Here's how the part is built. I have some questions about the finished solid (model axes, mm). Give positions to 0.01 mm unless a question says otherwise; leave off trailing zeros. Write each loop counter-clockwise with the first axis right and the second up, starting at its lowest first coordinate (ties: lowest second). Pieces come first, ordered by that corner, then holes. Notation, with made-up numbers: M 24,-30.75 L 75,-30.75 A10 cw 75,-15.75 Z; hole C 89.5,59 d7. An arc over 180 degrees is marked long. Answer as CSV lines item,"result". Start each with the question number.
Q1. For pin 1 (3 mm diameter, centred on x = 15.5, z = 490.5, fed in from -Y); pin 2 (2 mm diameter, centred on x = 16.5, z = 474.5, fed in from -Y); pin 3 (1.5 mm diameter, centred on x = 15.5, z = 470.5, fed in from -Y), each with a flat end and sliding along its axis, tell me the tip position at first contact or that it passes through.
Q2. Suppose I cut it at C-C (z = 475). Write out the boundary of the cut face in (x, y).
Q3. If I drill on line 1 along Y through (x, z) = (14.5, 498); line 2 along Y through (x, z) = (12.7, 466); line 3 along Z through (x, y) = (14.2, 2.5), over which ranges is the centre line in solid material (lowest first)?
Q4. Suppose I cut it at A-A (z = 469). Write out the boundary of the cut face in (x, y), then the cut area to 3 significant figures.
Q5. Suppose I cut it at B-B (x = 14.55). Write out the boundary of the cut face in (y, z), then the cut area to 3 significant figures.
Q6. Suppose I cut it at D-D (y = 19). Write out the boundary of the cut face in (x, z).
```python
from build123d import *

# Parameters (mm, degrees)
SKETCH1_R           = 2.2
SKETCH1_R_2         = 1.7
BOSS_EXTRUDE1_DEPTH = 5.08


with BuildPart() as part:
    # Sketch1 → Boss-Extrude1 (new body)
    with BuildSketch(Plane(origin=(17.497777778, 0, 0), x_dir=(0, 0, -1), z_dir=(1, 0, 0))):
        with BuildLine():
            Line((-499.600738517, 24.004018568), (-470.286926412, -0.333409807))
            ThreePointArc((-470.286926412, -0.333409807), (-464.654250247, 0.189045178), (-465.176705231, 5.821721344))
            Line((-465.176705231, 5.821721344), (-494.490517336, 30.159149718))
            ThreePointArc((-494.490517336, 30.159149718), (-500.123193502, 29.636694733), (-499.600738517, 24.004018568))
        make_face()
        with Locations((-467.731815822, 2.744155769)):
            Circle(SKETCH1_R, mode=Mode.SUBTRACT)
        with Locations((-497.045627927, 27.081584143)):
            Circle(SKETCH1_R_2, mode=Mode.SUBTRACT)
    extrude(amount=-BOSS_EXTRUDE1_DEPTH)


solid = part.part
```
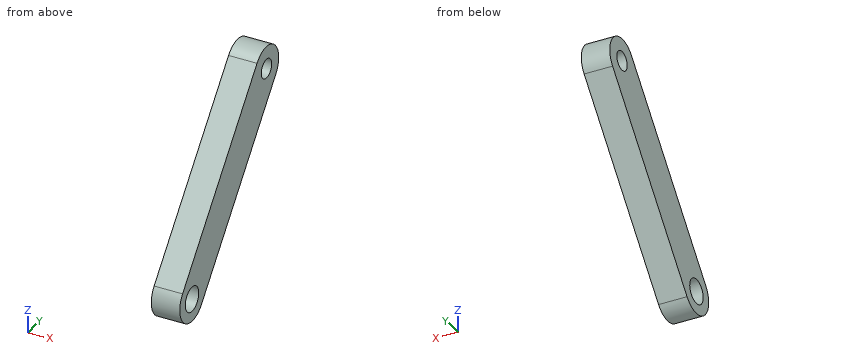
Resolved:
1,pin 1,"y = 15.2"
1,pin 2,"y = 2.33"
1,pin 3,"y = -0.71"
2,outline,"M 12.42,3.58 L 17.5,3.58 L 17.5,13.98 L 12.42,13.98 Z"
3,line 1,"22.68 to 25.67, 28.49 to 30.97"
3,line 2,"-0.86 to 1.39, 4.1 to 6.51"
3,line 3,"463.74 to 465.55, 469.92 to 473.7"
4,outline,"M 12.42,-1.05 L 17.5,-1.05 L 17.5,0.95 L 12.42,0.95 Z; M 12.42,4.54 L 17.5,4.54 L 17.5,9 L 12.42,9 Z"
4,area,"32.8 mm^2"
5,outline,"M -0.33,470.29 A4 ccw 5.82,465.18 L 30.16,494.49 A4 ccw 24,499.6 Z; hole C 2.74,467.73 d4.4; hole C 27.08,497.05 d3.4"
5,area,"331 mm^2"
6,outline,"M 12.42,481.05 L 17.5,481.05 L 17.5,493.57 L 12.42,493.57 Z"
